Part model, mm, in its own coordinate system. A direction names the side the tool comes from. Coordinates: 2 decimals unless noted, no trailing zeros. Write each loop counter-clockwise with the first axis right and the second up, starting at its lowest first coordinate (ties: lowest second). Pieces come first, ordered by that corner, then holes. Notation, with made-up numbers: M 29.5,-2 L 76.5,-2 A13 ccw 76.5,11 Z; hole C -27,42 d5. An arc over 180 degrees is marked long. Use a Markdown table: item, result. Add a question column.
Q1. Tool access for faces 1 (the flat face through (74.929, 3, 15)), 2 (the flat face through (-10, -2.968, 25)), 3 (the cylindrical face through (45.55, -0.05, 4.23)), 4 (the flat face through (-10, -8.668, 25)), 5 (the flat face through (10, -10, 23.9)): list every direction of +Z, -Z, +X, -X, +Y, -Y with a clear straight run to the whole face (end or side of a thin tool).
Q2. Slice it at A-A on z = 13.25. Write the cut outline in (x, y).
Q3. Slice it at B-B on y = 8.75. Write the cut outline in (x, z).
Q4. Wall check: L1, parallel to X at y = -0.5, z = 21.75; L2, parallel to Z at x = 29, y = 0.75; L3, parallel to Y at x = 59, z = 18. Give the ranges that are in metal, low to high. Write a range as from..to.
Q5. Slice it at C-C on x = 64. Write the cut outline in (y, z), then the cut area to 3 significant figures.
Q6. Pin check, flat tips, straight feed: pin 1 Ø1.6 at (x, y) = (55, -9.5) entering from +Z; pin 2 Ø1 at (y, z) = (-10, 26) entering from -X; pin 3 Ø9 at (x, y) = (22.5, 2.5) entering from +Z; pin 4 Ø5 at (x, z) = (7.5, 5) entering from +Y. Stop position of each tip, or through.
Q7. Mould opens along X. For faces 6 (the flat face through (76.929, 2, 13)), 7 (the cylindrical face through (14.02, -9.73, 13.3)), 8 (the flat face through (32, -10.668, 1)), 9 (the flat face through (44, 0, 5.5)) say: released by +X, released by -X, zero draft, split by the parting line, or undercut.
Q8. Slice it at D-D on y = -1.5. Write the cut outline in (x, z).
from build123d import *

# Parameters (mm, degrees)
ESBO_O1_W                = 87.854335153
ESBO_O1_H                = 25
RESSALTO_EXTRUS_O1_DEPTH = 3
ESBO_O1_11_R             = 4
ESBO_O1_11_R_2           = 2
RESSALTO_EXTRUS_O2_DEPTH = 5.5
ESBO_O1_12_W             = 1.938437843
ESBO_O1_12_H             = 5.7
ESBO_O1_12_H_2           = 9.6
ESBO_O1_12_W_2           = 9.7
ESBO_O1_12_H_3           = 2
ESBO_O1_12_W_3           = 2
RESSALTO_EXTRUS_O3_DEPTH = 23.9
ESBO_O1_13_W             = 1.938437843
ESBO_O1_13_H             = 5.7
ESBO_O1_13_W_2           = 9.7
ESBO_O1_13_H_2           = 2
ESBO_O1_13_W_3           = 2
RESSALTO_EXTRUS_O4_DEPTH = 26.9


with BuildPart() as part:
    # Esbo_o1 → Ressalto-extrus_o1 (new body)
    with BuildSketch(Plane.XY):
        with Locations((33.001638151, 1.832173033)):
            Rectangle(ESBO_O1_W, ESBO_O1_H)
    extrude(amount=RESSALTO_EXTRUS_O1_DEPTH)

    # Esbo_o1_11 → Ressalto-extrus_o2 (add)
    with BuildSketch(Plane.XY):
        with Locations((24.354470574, 1.482173033)):
            Circle(ESBO_O1_11_R)
        with Locations((24.354470574, 1.482173033)):
            Circle(ESBO_O1_11_R_2, mode=Mode.SUBTRACT)
        with Locations((41.854470574, 1.482173033)):
            Circle(ESBO_O1_11_R)
        with Locations((41.854470574, 1.482173033)):
            Circle(ESBO_O1_11_R_2, mode=Mode.SUBTRACT)
    extrude(amount=RESSALTO_EXTRUS_O2_DEPTH)

    # Esbo_o1_12 → Ressalto-extrus_o3 (add)
    with BuildSketch(Plane.XY):
        with BuildLine():
            ThreePointArc((-8.987091583, 12.332173033), (-8.9716974, 13.332646658), (-8.925529426, 14.332173033))
            Line((-8.925529426, 14.332173033), (-10.925529426, 14.332173033))
            Line((-10.925529426, 14.332173033), (-10.925529426, 12.332173033))
            Line((-10.925529426, 12.332173033), (-8.987091583, 12.332173033))
        make_face()
        with Locations((-9.956310504, 9.482173033)):
            Rectangle(ESBO_O1_12_W, ESBO_O1_12_H)
        with Locations((-9.956310504, 1.832173033)):
            Rectangle(ESBO_O1_12_W, ESBO_O1_12_H_2)
        Polygon((-10.925529426, -8.667826967), (-8.987091583, -8.667826967), (-8.987091583, -6.667826967), (-8.987091583, -2.967826967), (-10.925529426, -2.967826967), align=None)
        Polygon((-8.925529426, -10.667826967), (-2.625529426, -10.667826967), (-2.625529426, -8.667826967), (-8.987091583, -8.667826967), (-10.925529426, -8.667826967), (-10.925529426, -10.667826967), align=None)
        with Locations((2.224470574, -9.667826967)):
            Rectangle(ESBO_O1_12_W_2, ESBO_O1_12_H_3)
        with BuildLine():
            Line((7.074470574, -10.667826967), (15.138180648, -10.667826967))
            ThreePointArc((15.138180648, -10.667826967), (14.007108736, -9.720264336), (12.972906533, -8.667826967))
            Line((12.972906533, -8.667826967), (7.074470574, -8.667826967))
            Line((7.074470574, -8.667826967), (7.074470574, -10.667826967))
        make_face()
        with BuildLine():
            ThreePointArc((53.236034614, -8.667826967), (52.201832411, -9.720264336), (51.0707605, -10.667826967))
            Line((51.0707605, -10.667826967), (54.381392228, -10.667826967))
            Line((54.381392228, -10.667826967), (58.928805727, -10.667826967))
            Line((58.928805727, -10.667826967), (58.928805727, -8.667826967))
            Line((58.928805727, -8.667826967), (53.236034614, -8.667826967))
        make_face()
        with Locations((63.778805727, -9.667826967)):
            Rectangle(ESBO_O1_12_W_2, ESBO_O1_12_H_3)
        Polygon((68.628805727, -8.667826967), (68.628805727, -10.667826967), (76.928805727, -10.667826967), (76.928805727, -8.667826967), (74.928805727, -8.667826967), align=None)
        with Locations((75.928805727, -5.817826967)):
            Rectangle(ESBO_O1_12_W_3, ESBO_O1_12_H)
        with Locations((75.928805727, 1.832173033)):
            Rectangle(ESBO_O1_12_W_3, ESBO_O1_12_H_2)
        with Locations((75.928805727, 9.482173033)):
            Rectangle(ESBO_O1_12_W_3, ESBO_O1_12_H)
        with Locations((75.928805727, 13.332173033)):
            Rectangle(ESBO_O1_12_W_3, ESBO_O1_12_H_3)
    extrude(amount=RESSALTO_EXTRUS_O3_DEPTH)

    # Esbo_o1_13 → Ressalto-extrus_o4 (add)
    with BuildSketch(Plane.XY):
        with Locations((-9.956310504, 9.482173033)):
            Rectangle(ESBO_O1_13_W, ESBO_O1_13_H)
        Polygon((-10.925529426, -8.667826967), (-8.987091583, -8.667826967), (-8.987091583, -6.667826967), (-8.987091583, -2.967826967), (-10.925529426, -2.967826967), align=None)
        with Locations((2.224470574, -9.667826967)):
            Rectangle(ESBO_O1_13_W_2, ESBO_O1_13_H_2)
        with Locations((63.778805727, -9.667826967)):
            Rectangle(ESBO_O1_13_W_2, ESBO_O1_13_H_2)
        with Locations((75.928805727, 9.482173033)):
            Rectangle(ESBO_O1_13_W_3, ESBO_O1_13_H)
        with Locations((75.928805727, -5.817826967)):
            Rectangle(ESBO_O1_13_W_3, ESBO_O1_13_H)
    extrude(amount=RESSALTO_EXTRUS_O4_DEPTH)


solid = part.part
Recorded:
| question | item | result |
|---|---|---|
| 1 | face 1 | +Z, +Y |
| 1 | face 2 | +Z, +X, -X |
| 1 | face 3 | +Z |
| 1 | face 4 | +Z, -X, -Y |
| 1 | face 5 | +Z, +Y, -Y |
| 2 | outline | M -10.93,-10.67 L 15.14,-10.67 A15.25 cw 12.97,-8.67 L -8.99,-8.67 L -8.99,12.33 A32.52 cw -8.93,14.33 L -10.93,14.33 Z; M 51.07,-10.67 L 76.93,-10.67 L 76.93,14.33 L 74.93,14.33 L 74.93,-8.67 L 53.24,-8.67 A15.25 cw Z |
| 3 | outline | M -10.93,0 L 76.93,0 L 76.93,26.9 L 74.93,26.9 L 74.93,3 L -8.99,3 L -8.99,26.9 L -10.93,26.9 Z |
| 4 | L1 | -10.93..-8.99, 74.93..76.93 |
| 4 | L2 | 0..3 |
| 4 | L3 | -10.67..-8.67 |
| 5 | outline | M -10.67,0 L 14.33,0 L 14.33,3 L -8.67,3 L -8.67,26.9 L -10.67,26.9 Z |
| 5 | area | 123 mm² |
| 6 | pin 1 | z = 23.9 |
| 6 | pin 2 | x = -2.63 |
| 6 | pin 3 | z = 5.5 |
| 6 | pin 4 | y = 14.33 |
| 7 | face 6 | released by +X |
| 7 | face 7 | undercut |
| 7 | face 8 | zero draft |
| 7 | face 9 | undercut |
| 8 | outline | M -10.93,0 L 76.93,0 L 76.93,23.9 L 74.93,23.9 L 74.93,3 L 44.52,3 L 44.52,5.5 L 39.19,5.5 L 39.19,3 L 27.02,3 L 27.02,5.5 L 21.69,5.5 L 21.69,3 L -8.99,3 L -8.99,23.9 L -10.93,23.9 Z |
